Could you check a few things on this model? Use its own coordinates, in mm. A direction names the side the tool comes from. Give positions to 0.01 mm unless a question says otherwise; leave off trailing zeros. Loops run counter-clockwise (first coordinate to the right, second up) from the corner with the lowest first, then second, coordinate; pieces in that order, holes last. Notation, with made-up numbers: (14, 4.5) - (71, 4.5) arc R27 cw to (71, 39.5) - close; hole circle Ø4 at (53.5, -36). An arc over 180 degrees is marked (long way). One line per item, written item: value. Start each with the question number.
Q1. For faces 1 (the face through (-3, -15, 8)), 2 (the face through (3.825, 12, 28)), 3 (the face through (3, -12, 48.55)), 4 (the face through (11.255, 8.981, 38.318)), 5 (the face through (-6.364, -6, 51)), which set-ups out of +Z, -Z, +X, -X, +Y, -Y let a thin tool reach every point of the face, with its end or its side?
Q2. I want a section at C-C (z = 17.5). Please give me the cut outline in (x, y) (1 decimal), then the cut area to 3 significant figures.
Q3. I want a section at A-A (y = 0). Count the separate pieces of the cut face and the enclosed holes in it, then the cut area to 3 significant figures.
Q4. If we mould it in two halves opening along Z, with no side actions, what happens to faces 6 (the face through (0, 14, 9)), 7 (the face through (11.255, -19.399, 52.606)), 8 (the face through (2, -6, 46.55))? For each: released by +Z, released by -Z, zero draft, split by the parting line, or undercut.
Q5. I want a section at B-B (x = -2). Please give me the cut outline in (y, z), then the cut area to 3 significant figures.
Q6. I'm going to push flat-ended pins straight in: P1, Ø1.6, axis at x = 3, y = -11.5, coming from the +Z side; P2, Ø3.5, axis at y = -12, z = 28.275, coming from the +X side; P3, Ø2.5, axis at x = -0.5, y = 15, coming from the -Z side. Where does each tip first touch, or does it pass through?
Q7. If I drill on line 1 (Y direction, x = 0, z = 2); line 2 (X direction, y = -7.5, z = 24) (1 decimal); line 3 (X direction, y = 14, z = 4) (3 decimals), over which ranges is the centre line in solid material (lowest first)? Write a range as from..to.
```python
from build123d import *

# Parameters (mm, degrees)
SKETCH1_W           = 23.65
SKETCH1_H           = 40
BOSS_EXTRUDE1_DEPTH = 56.55
SKETCH2_W           = 16
SKETCH2_H           = 28.38
CUT_EXTRUDE1_DEPTH  = 62.137002911
SKETCH3_R           = 7
CUT_EXTRUDE2_DEPTH  = 6.2205
SKETCH6_R           = 3.025
CUT_EXTRUDE4_DEPTH  = 8
SKETCH4_W           = 11.968
SKETCH4_H           = 10
BOSS_EXTRUDE2_DEPTH = 28.38
SKETCH5_W           = 12.292
SKETCH5_H           = 28.38
CUT_EXTRUDE3_DEPTH  = 6.2205
FILLET5_R           = 2
SKETCH9_W           = 8
SKETCH9_H           = 11
BOSS_EXTRUDE3_DEPTH = 16
SKETCH8_R           = 2.7
CUT_EXTRUDE6_DEPTH  = 9
SKETCH7_R           = 2.7
CUT_EXTRUDE5_DEPTH  = 8
FILLET4_R           = 2
FILLET8_R           = 1


with BuildPart() as part:
    # Sketch1 → Boss-Extrude1 (new body)
    with BuildSketch(Plane.XY):
        Rectangle(SKETCH1_W, SKETCH1_H)
    extrude(amount=BOSS_EXTRUDE1_DEPTH)

    # Sketch2 → Cut-Extrude1 (cut, through all)
    with BuildSketch(Plane.XY.offset(56.55)):
        with Locations((-2.3955, -5.81)):
            Rectangle(SKETCH2_W, SKETCH2_H)
    extrude(amount=-CUT_EXTRUDE1_DEPTH, mode=Mode.SUBTRACT)

    # Sketch3 → Cut-Extrude2 (cut)
    with BuildSketch(Plane(origin=(11.825, 0, 0), x_dir=(0, 0, -1), z_dir=(1, 0, 0))):
        with Locations(Location((-28.275, 0, 0), (0, 0, 90))):
            Circle(SKETCH3_R)
    extrude(amount=-CUT_EXTRUDE2_DEPTH, mode=Mode.SUBTRACT)

    # Sketch6 → Cut-Extrude4 (cut)
    with BuildSketch(Plane(origin=(11.825, 0, 0), x_dir=(0, 0, -1), z_dir=(1, 0, 0))):
        with Locations(Location((-28.275, 12, 0), (0, 0, 90))):
            Circle(SKETCH6_R)
        with Locations(Location((-28.275, -12, 0), (0, 0, 90))):
            Circle(SKETCH6_R)
    extrude(amount=-CUT_EXTRUDE4_DEPTH, mode=Mode.SUBTRACT)

    # Sketch4 → Boss-Extrude2 (add)
    with BuildSketch(Plane.XZ.offset(-8.38)):
        with Locations((-0.3795, 51.55)):
            Rectangle(SKETCH4_W, SKETCH4_H)
    extrude(amount=BOSS_EXTRUDE2_DEPTH)

    # Sketch5 → Cut-Extrude3 (cut)
    with BuildSketch(Plane(origin=(11.825, 0, 0), x_dir=(0, 0, -1), z_dir=(1, 0, 0))):
        with Locations((-40.404, -5.81)):
            Rectangle(SKETCH5_W, SKETCH5_H)
    extrude(amount=-CUT_EXTRUDE3_DEPTH, mode=Mode.SUBTRACT)

    # Fillet5
    fillet5_edges = [part.edges().sort_by_distance(p)[0] for p in [
        (5.6045, 8.38, 17.129),
    ]]
    fillet(fillet5_edges, radius=FILLET5_R)

    # Sketch9 → Boss-Extrude3 (add)
    with BuildSketch(Plane(origin=(-10.3955, 0, 0), x_dir=(0, 0, -1), z_dir=(1, 0, 0))):
        with Locations((-4, -14.5)):
            Rectangle(SKETCH9_W, SKETCH9_H)
    extrude(amount=BOSS_EXTRUDE3_DEPTH)

    # Sketch8 → Cut-Extrude6 (cut)
    with BuildSketch(Plane(origin=(0, 0, 0), x_dir=(-1, 0, 0), z_dir=(0, 0, -1))):
        with Locations((0, 14.19)):
            Circle(SKETCH8_R)
        with Locations((0, -14.5)):
            Circle(SKETCH8_R)
    extrude(amount=-CUT_EXTRUDE6_DEPTH, mode=Mode.SUBTRACT)

    # Sketch7 → Cut-Extrude5 (cut)
    with BuildSketch(Plane.XY.offset(56.55)):
        with Locations((2.73075, 12.5)):
            Circle(SKETCH7_R)
        with Locations((2.73075, -12.5)):
            Circle(SKETCH7_R)
    extrude(amount=-CUT_EXTRUDE5_DEPTH, mode=Mode.SUBTRACT)

    # Fillet4
    fillet4_edges = [part.edges().sort_by_distance(p)[0] for p in [
        (5.6045, -14.5, 8),
        (5.6045, -9, 4),
        (2.73075, -20, 46.55),
        (2.73075, 8.38, 46.55),
        (8.71475, 3.633691099, 34.258),
        (8.71475, -3.633691099, 34.258),
        (11.825, -20, 17.129),
        (11.825, 8.38, 40.404),
        (11.825, -11.816845549, 34.258),
        (11.825, 6.006845549, 34.258),
        (11.825, -5.81, 46.55),
        (8.71475, -20, 34.258),
        (11.825, -20, 51.55),
        (11.825, 20, 28.275),
    ]]
    fillet(fillet4_edges, radius=FILLET4_R)

    # Fillet8
    fillet8_edges = [part.edges().sort_by_distance(p)[0] for p in [
        (-10.3955, -14.5, 8),
        (-10.3955, -9, 4),
        (-10.3955, 8.38, 28.275),
        (-6.3635, 8.38, 50.55),
    ]]
    fillet(fillet8_edges, radius=FILLET8_R)


solid = part.part
```
Worked answers:
1. face 1: -Y
1. face 2: +X
1. face 3: +Z
1. face 4: +X, -Y
1. face 5: +Z, -Y
2. outline: (-11.8, -20) - (-10.4, -20) - (-10.4, 7.4) arc R1 cw to (-9.4, 8.4) - (3.6, 8.4) arc R2 cw to (5.6, 6.4) - (5.6, -20) - (9.8, -20) arc R2 ccw to (11.8, -18) - (11.8, 18) arc R2 ccw to (9.8, 20) - (-11.8, 20) - close
2. area: 491 mm²
3. separate pieces: 3
3. enclosed holes: 0
3. area: 394 mm²
4. face 6: released by -Z
4. face 7: zero draft
4. face 8: undercut
5. outline: (-20, 0) - (-16.31, 0) - (-16.31, 8) - (-20, 8) - close; (-20, 48.55) arc R2 ccw to (-18, 46.55) - (6.38, 46.55) arc R2 cw to (8.38, 44.55) - (8.38, 0) - (12.38, 0) - (12.38, 9) - (16, 9) - (16, 0) - (20, 0) - (20, 56.55) - (-20, 56.55) - close; (-12.69, 0) - (-9, 0) - (-9, 8) - (-12.69, 8) - close
5. area: 967 mm²
6. P1: stops at z = 48.55
6. P2: stops at x = -10.4
6. P3: stops at z = 9
7. line 1: y = -20..-17.2, -11.8..-9, 8.38..11.49, 16.89..20
7. line 2: x = -11.8..-10.4, 5.6..11.8
7. line 3: x = -11.825..-2.693, 2.693..11.825
